For this review, take the finished solid that the model builds, in its own axes (mm). Face numbers are marked on the shaded views. A direction names the side the tool comes from. Coordinates: 2 decimals unless noted, no trailing zeros. Loops run counter-clockwise (first coordinate to the right, second up) from the corner with the lowest first, then second, coordinate; pieces in that order, holes last. Notation, with made-up numbers: (84, 46.25) -> (123, 46.25) arc R23 cw to (123, 82.25) -> close; hole circle Ø5 at (52.25, -3.5). An arc over 180 degrees is marked (long way). Use a Markdown table: item, result.
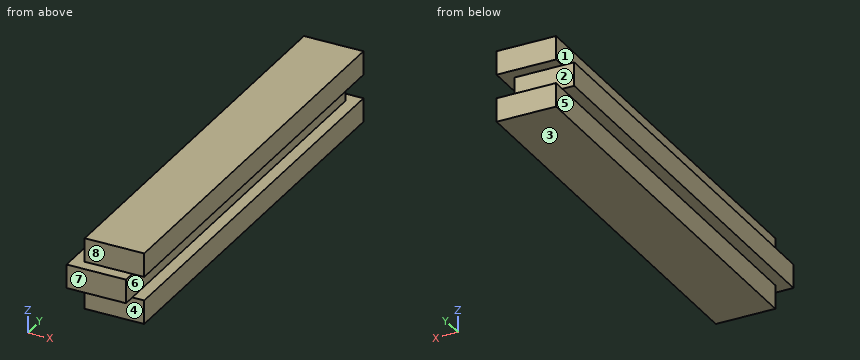
from build123d import *

# Parameters (mm, degrees)
F2_W     = 7.9375
F2_H     = 55.5625
F3_DEPTH = 3.175
F4_W     = 7.9375
F4_H     = 55.5625
F5_DEPTH = 3.175
F6_W     = 7.9375
F6_H     = 55.5625
F7_DEPTH = 3.175


# Not quite as in the source:
# - a variable given as a bare number and used for a length is read in inches; the dataset says mm whatever the document's units were


with BuildPart() as f3:
    # F2 (on Top) → F3 (new body)
    with BuildSketch(Plane.XY):
        with Locations((3.96875, 27.78125)):
            Rectangle(F2_W, F2_H)
    extrude(amount=F3_DEPTH)

    # F4 (on face) → F5 (join)
    with BuildSketch(Plane.XY.offset(3.175)):
        with Locations((2.38125, 26.19375)):
            Rectangle(F4_W, F4_H)
    extrude(amount=F5_DEPTH)

    # F6 (on face) → F7 (join)
    with BuildSketch(Plane.XY.offset(6.35)):
        with Locations((3.96875, 27.78125)):
            Rectangle(F6_W, F6_H)
    extrude(amount=F7_DEPTH)


solid = f3.part
(1) For line 1 along Z through (x, y) = (6.75, 32.5) (3 decimals); line 2 along X through (y, z) = (14.5, 4.75); line 3 along X through (y, z) = (16.5, 1.5), list the stretches that pass through material, from the lowest coordinate up.
Found:
| item | result |
|---|---|
| line 1 | z = 0 to 3.175, 6.35 to 9.525 |
| line 2 | x = -1.59 to 6.35 |
| line 3 | x = 0 to 7.94 |
(2) Take a section at D-D on z = 1.5. Write out the cut boundary in (x, y).
Found:
| item | result |
|---|---|
| outline | (0, 0) -> (7.94, 0) -> (7.94, 55.56) -> (0, 55.56) -> close |
(3) Mouldability with a two-part tool opening along Z and no side actions: class the marked faces 1, 2 and 3 as pulls with the +Z half, pulls with the -Z half, needs draft (parallel to the pull), parting line crosses it, or undercut.
Found:
| item | result |
|---|---|
| face 1 | needs draft |
| face 2 | undercut |
| face 3 | pulls with the -Z half |
(4) For the marked faces 4, 5, 6, 7 and 8, list the 3-axis set-ups (+Z, -Z, +X, -X, +Y, -Y) from which the entire face can be reached by the end or side of a thin tool; tool diameter is ignored.
Found:
| item | result |
|---|---|
| face 4 | -Z, +X, -X, -Y |
| face 5 | -Z, -X, +Y, -Y |
| face 6 | +X, +Y, -Y |
| face 7 | +Z, -Z, +X, -X, -Y |
| face 8 | +Z, +X, -X, -Y |
(5) For pin 1 Ø1 at (y, z) = (27.5, 7.5) entering from -X; pin 2 Ø1.6 at (x, z) = (6, 1.5) entering from -Y; pin 3 Ø1.6 at (y, z) = (16.5, 5.5) entering from +X, all flat-tipped, find the tip position at first contact; note any pin that passes through.
Found:
| item | result |
|---|---|
| pin 1 | stops at x = 0 |
| pin 2 | stops at y = 0 |
| pin 3 | stops at x = 6.35 |
